Verification items for the finished model (mm, model axes). Coordinates: 2 decimals unless noted, no trailing zeros. Write each loop counter-clockwise with the first axis right and the second up, starting at its lowest first coordinate (ties: lowest second). Pieces come first, ordered by that corner, then holes. Notation, with made-up numbers: (60.5, -25) -> (71.5, -25) arc R15 ccw to (71.5, -6) -> close; hole circle Ø3 at (1.25, 9.5). An arc over 180 degrees is marked (long way). Write each question's results on one line, items separated by ' | '. Start each with the question number.
from build123d import *

# Parameters (mm, degrees)
EXTRUDE_1_DEPTH     = 12
CUT_EXTRUDE_START   = -2
CUT_EXTRUDE_1_DEPTH = 6
CHAMFER_1_SIZE      = 7
CUT_EXTRUDE_2_DEPTH = 6


with BuildPart() as part:
    # 草图1 → 凸台-拉伸1 (new body)
    with BuildSketch(Plane.XY):
        Polygon((0, 12), (0, -12), (587, -12), (611, 12), align=None)
    extrude(amount=EXTRUDE_1_DEPTH)

    # 草图2 → 切除-拉伸1 (cut)
    with BuildSketch(Plane.XY.offset(12).offset(CUT_EXTRUDE_START)):
        Polygon((278.5, 12), (285, 5.5), (325, 5.5), (331.5, 12), align=None)
    cut_extrude_1 = extrude(amount=-CUT_EXTRUDE_1_DEPTH, mode=Mode.SUBTRACT)

    # 倒角1
    chamfer_1_edges = [part.edges().sort_by_distance(p)[0] for p in [
        (0, 0, 12),
    ]]
    chamfer(chamfer_1_edges, length=CHAMFER_1_SIZE)

    # 镜向1: 切除-拉伸1 across plane
    add(cut_extrude_1.mirror(Plane.ZX), mode=Mode.SUBTRACT)

    # 草图3 → 切除-拉伸2 (cut)
    with BuildSketch(Plane.XY.offset(12).offset(CUT_EXTRUDE_START)):
        Polygon((593.5, -5.5), (587, -12), (557.5, -12), (564, -5.5), align=None)
        Polygon((611, 12), (604.5, 5.5), (564, 5.5), (557.5, 12), align=None)
        Polygon((0, 12), (0, 5.5), (45, 5.5), (51.5, 12), align=None)
        Polygon((0, -12), (0, -5.5), (45, -5.5), (51.5, -12), align=None)
    extrude(amount=-CUT_EXTRUDE_2_DEPTH, mode=Mode.SUBTRACT)


solid = part.part
1. Sectioned sample at A-A on z = 7.5. Record the cut outline in (x, y).
2. Sectioned sample at C-C on x = 296. Record the cut outline in (y, z), plus the area to 3 significant figures.
3. Sectioned sample at B-B on y = -0.75. Record the cut outline in (x, z), plus the area to 3 significant figures.
4. Depth check by flat-ended pin: pin 1 Ø1 at (y, z) = (-9.5, 10.5) entering from +X; pin 2 Ø1.8 at (x, z) = (576, 6) entering from +Y. Enter the tip coordinate at first touch or a pass-through.
5. Material ranges on probe 1 along Y at (x, z) = (293, 4.5); probe 2 along X at (y, z) = (6.75, 4.5); probe 3 along X at (y, z) = (7, 4.75), recorded low to high. Write a range as from..to.
Computed values:
1) outline: (2.5, -5.5) -> (45, -5.5) -> (51.5, -12) -> (278.5, -12) -> (285, -5.5) -> (325, -5.5) -> (331.5, -12) -> (557.5, -12) -> (564, -5.5) -> (593.5, -5.5) -> (604.5, 5.5) -> (564, 5.5) -> (557.5, 12) -> (331.5, 12) -> (325, 5.5) -> (285, 5.5) -> (278.5, 12) -> (51.5, 12) -> (45, 5.5) -> (2.5, 5.5) -> close
2) outline: (-12, 0) -> (12, 0) -> (12, 4) -> (5.5, 4) -> (5.5, 10) -> (12, 10) -> (12, 12) -> (-12, 12) -> (-12, 10) -> (-5.5, 10) -> (-5.5, 4) -> (-12, 4) -> close | area: 210 mm^2
3) outline: (0, 0) -> (598.25, 0) -> (598.25, 12) -> (7, 12) -> (0, 5) -> close | area: 7,150 mm^2
4) pin 1: stops at x = 590 | pin 2: stops at y = 5.5
5) probe 1: y = -5.5..5.5 | probe 2: x = 46.25..283.75, 326.25..562.75 | probe 3: x = 46.5..283.5, 326.5..562.5
